Read the model definition and answer for the solid it produces. Units are mm, in the model's axes. Give positions to 0.01 mm unless a question says otherwise; leave off trailing zeros. Order: outer loops, then holes, each group sorted by start corner. A loop starts at its lowest first (then second) coordinate and runs counter-clockwise, first axis right, second up. Notation, with made-up numbers: (38.5, 44) -> (94.5, 44) arc R25 ccw to (94.5, 59) -> close; hole circle Ø9 at (11, 33). An arc over 180 degrees is marked (long way). One line per question, with ' | ' between items. Start each with the question number.
```python
from build123d import *

# Parameters (mm, degrees)
SKETCH1_W               = 30
SKETCH1_H               = 25
BOSS_EXTRUDE1_DEPTH     = 5
CUT_EXTRUDE1_REACH      = 22.156
SKETCH2_R               = 1.6
CUT_EXTRUDE2_DEPTH      = 21.155644371
CUT_EXTRUDE2_DEPTH_BACK = 5


with BuildPart() as part:
    # Sketch1 → Boss-Extrude1 (new body)
    with BuildSketch(Plane.XY):
        Rectangle(SKETCH1_W, SKETCH1_H)
    extrude(amount=BOSS_EXTRUDE1_DEPTH)

    # Sketch2 → Cut-Extrude1 (cut, up to next)
    with BuildSketch(Plane.XY.offset(5), mode=Mode.PRIVATE) as cut_extrude1_sk1:
        with Locations((-10, -7.5)):
            Circle(SKETCH2_R)
    cut_extrude1_tool1 = extrude(cut_extrude1_sk1.sketch, amount=-CUT_EXTRUDE1_REACH, mode=Mode.PRIVATE) & part.part
    # Sketch2 → Cut-Extrude1 (cut, up to next)
    with BuildSketch(Plane.XY.offset(5), mode=Mode.PRIVATE) as cut_extrude1_sk2:
        with Locations((0, -7.5)):
            Circle(SKETCH2_R)
    cut_extrude1_tool2 = extrude(cut_extrude1_sk2.sketch, amount=-CUT_EXTRUDE1_REACH, mode=Mode.PRIVATE) & part.part
    # Sketch2 → Cut-Extrude1 (cut, up to next)
    with BuildSketch(Plane.XY.offset(5), mode=Mode.PRIVATE) as cut_extrude1_sk3:
        with Locations((10, -7.5)):
            Circle(SKETCH2_R)
    cut_extrude1_tool3 = extrude(cut_extrude1_sk3.sketch, amount=-CUT_EXTRUDE1_REACH, mode=Mode.PRIVATE) & part.part
    # Sketch2 → Cut-Extrude1 (cut, up to next)
    with BuildSketch(Plane.XY.offset(5), mode=Mode.PRIVATE) as cut_extrude1_sk4:
        with Locations((-10, 7.5)):
            Circle(SKETCH2_R)
    cut_extrude1_tool4 = extrude(cut_extrude1_sk4.sketch, amount=-CUT_EXTRUDE1_REACH, mode=Mode.PRIVATE) & part.part
    add(cut_extrude1_tool1.solids().sort_by_distance((-10, -7.5, 5))[0], mode=Mode.SUBTRACT)
    add(cut_extrude1_tool2.solids().sort_by_distance((0, -7.5, 5))[0], mode=Mode.SUBTRACT)
    add(cut_extrude1_tool3.solids().sort_by_distance((10, -7.5, 5))[0], mode=Mode.SUBTRACT)
    add(cut_extrude1_tool4.solids().sort_by_distance((-10, 7.5, 5))[0], mode=Mode.SUBTRACT)

    # Sketch3 → Cut-Extrude2 (cut, two sides: drawn at the far end of the back side and taken through both)
    with BuildSketch(Plane.XY.offset(5).offset(-CUT_EXTRUDE2_DEPTH_BACK)):
        Polygon((-68.5998728, 52.2499205), (-5, 12.5), (15, 0), (78.5998728, -39.7499205), (158.099713801, 87.449825101), (10.8999682, 179.449666101), align=None)
    extrude(amount=CUT_EXTRUDE2_DEPTH + CUT_EXTRUDE2_DEPTH_BACK, mode=Mode.SUBTRACT)


solid = part.part
```
Q1. Given P1, Ø4, axis at x = 7, y = 9, coming from the +Z side; P2, Ø1.5, axis at x = 6.5, z = 4, coming from the +Y side, each flat-ended and moving along its own axis, determine where each tip first touches the part or whether it passes through.
Q2. A cutting plane is placed at B-B, the plane z = 2.85. Determine the outline of the cut face in (x, y), then the cut area to 3 significant figures.
Q3. A cutting plane is placed at D-D, the plane x = 0. Determine the outline of the cut face in (y, z) (3 decimals).
Q4. Determine the mould class of faces 1 (the flat face through (-10, 12.5, 2)), 2 (the cylindrical face through (-11.27, -8.47, 2.54)), 3 (the flat face through (0, -3, 0)) for opening direction Y: pulls with the +Y half, pulls with the -Y half, needs draft (parallel to the pull), parting line crosses it, or undercut.
Q5. A cutting plane is placed at C-C, the plane y = -7.5. Determine the outline of the cut face in (x, z), then the cut area to 3 significant figures.
Q6. Find the intervals of material crossed by line 1 (Y direction, x = -10, z = 3.2); line 2 (Y direction, x = 7, z = 0.65); line 3 (Y direction, x = 9, z = 2.6), in increasing order.
Q7. A cutting plane is placed at A-A, the plane y = 7.5. Determine the outline of the cut face in (x, z), then the cut area to 3 significant figures.
Geometry results:
1) P1: through | P2: y = 5.78
2) outline: (-15, -12.5) -> (15, -12.5) -> (15, 0) -> (-5, 12.5) -> (-15, 12.5) -> close; hole circle Ø3.2 at (-10, -7.5); hole circle Ø3.2 at (-10, 7.5); hole circle Ø3.2 at (0, -7.5); hole circle Ø3.2 at (10, -7.5) | area: 593 mm²
3) outline: (-12.5, 0) -> (-9.1, 0) -> (-9.1, 5) -> (-12.5, 5) -> close; (-5.9, 0) -> (9.375, 0) -> (9.375, 5) -> (-5.9, 5) -> close
4) face 1: pulls with the +Y half | face 2: undercut | face 3: needs draft
5) outline: (-15, 0) -> (-11.6, 0) -> (-11.6, 5) -> (-15, 5) -> close; (-8.4, 0) -> (-1.6, 0) -> (-1.6, 5) -> (-8.4, 5) -> close; (1.6, 0) -> (8.4, 0) -> (8.4, 5) -> (1.6, 5) -> close; (11.6, 0) -> (15, 0) -> (15, 5) -> (11.6, 5) -> close | area: 102 mm²
6) line 1: -12.5 to -9.1, -5.9 to 5.9, 9.1 to 12.5 | line 2: -12.5 to 5 | line 3: -12.5 to -8.75, -6.25 to 3.75
7) outline: (-15, 0) -> (-11.6, 0) -> (-11.6, 5) -> (-15, 5) -> close; (-8.4, 0) -> (3, 0) -> (3, 5) -> (-8.4, 5) -> close | area: 74.0 mm²
